from build123d import *

# Parameters (mm, degrees)
F0_W     = 61
F0_H     = 42
F0_W_2   = 28
F0_H_2   = 3.6
F0_R     = 6.5
F0_R_2   = 13.35
F0_R_3   = 11.75
F1_DEPTH = 1.2
F2_DEPTH = 10
F3_DEPTH = 5
F4_W     = 22.4
F4_H     = 2.5
F5_DEPTH = 5


with BuildPart() as f1:
    # F0 (on Top) → F1 (new body)
    with BuildSketch(Plane.XY):
        with Locations((30.5, 21)):
            Rectangle(F0_W, F0_H)
        with Locations((24, 7.8)):
            Rectangle(F0_W_2, F0_H_2, mode=Mode.SUBTRACT)
        with Locations((12.5, 28.3)):
            Circle(F0_R, mode=Mode.SUBTRACT)
        with Locations((44.25, 26.15)):
            Circle(F0_R_2, mode=Mode.SUBTRACT)
        with Locations((44.25, 26.15)):
            Circle(F0_R_2)
        with Locations((44.25, 26.15)):
            Circle(F0_R_3, mode=Mode.SUBTRACT)
    extrude(amount=F1_DEPTH)

    # F0 (on Top) → F2 (join)
    with BuildSketch(Plane.XY):
        with Locations((44.25, 26.15)):
            Circle(F0_R_2)
        with Locations((44.25, 26.15)):
            Circle(F0_R_3, mode=Mode.SUBTRACT)
    extrude(amount=F2_DEPTH)

    # F0 (on Top) → F3 (join)
    with BuildSketch(Plane.XY):
        with Locations((24, 7.8)):
            Rectangle(F0_W_2, F0_H_2)
    extrude(amount=F3_DEPTH)

    # F4 (on face) → F5 (cut)
    with BuildSketch(Plane.XZ.offset(-6)):
        with Locations((24, 2.45)):
            Rectangle(F4_W, F4_H)
    extrude(amount=-F5_DEPTH, mode=Mode.SUBTRACT)


solid = f1.part
Geometry check sheet. Reference: the model listing, model coordinates, mm. A direction names the side the tool comes from. Give positions to 0.01 mm unless a question says otherwise; leave off trailing zeros. Write each loop counter-clockwise with the first axis right and the second up, starting at its lowest first coordinate (ties: lowest second). Pieces come first, ordered by that corner, then holes. Notation, with made-up numbers: M -39.75,39.5 L -24.75,39.5 A10 cw -24.75,44.5 Z; hole C 34.25,-37.75 d7. An arc over 180 degrees is marked long. Answer as CSV lines item,"result". Start each with the question number.
Q1. Section check D-D, the plane x = 14. Record the cut outline in (y, z).
Q2. Tool access check on faces 1 (the face through (56.984, 30.16, 5.538)), 2 (the face through (24, 8, 3.7)), 3 (the face through (12.8, 8, 2)), 4 (the face through (24, 8, 5)). Record the directions out of +Z, -Z, +X, -X, +Y, -Y that give a thin tool (end or side, any length) a straight path to the whole face; none if there is none.
Q3. Section check C-C, the plane z = 8. Record the cut outline in (x, y), then the cut area to 3 significant figures.
Q4. Section check A-A, the plane y = 28.3. Record the cut outline in (x, z).
Q5. Release check for a two-part mould opening along Y. For faces 5 (the face through (32.51, 26.67, 4.93)), 6 (the face through (30, 21, 0)), 7 (the face through (30, 0, 1)) record: pulls with the +Y half, pulls with the -Y half, needs draft (parallel to the pull), parting line crosses it, or undercut.
Q6. Go/stop test with flat-tipped pins: pin 1 (1.5 mm diameter, centred on y = 14, z = 7.5, fed in from -X); pin 2 (15 mm diameter, centred on x = 12.5, y = 28.3, fed in from +Z); pin 3 (14 mm diameter, centred on x = 44.25, y = 26.15, fed in from -Z); pin 4 (3 mm diameter, centred on x = 20, z = 4, fed in from -Y). Record where each tip stops, or that it passes through.
Q7. Section check B-B, the plane x = 44.25. Record the cut outline in (y, z).
Q8. Material ranges on L1, parallel to Y at x = 12.5, z = 0.8; L2, parallel to Z at x = 14.5, y = 7.5; L3, parallel to Y at x = 44, z = 8.25, recorded low to high.
Geometry says:
1,outline,"M 0,0 L 21.98,0 L 21.98,1.2 L 0,1.2 Z; M 6,3.7 L 9.6,3.7 L 9.6,5 L 6,5 Z; M 34.62,0 L 42,0 L 42,1.2 L 34.62,1.2 Z"
2,face 1,"+Z"
2,face 2,"-Y"
2,face 3,"+Y, -Y"
2,face 4,"+Z, +X, -X, -Y"
3,outline,"C 44.25,26.15 d26.7; hole C 44.25,26.15 d23.5"
3,area,"126 mm^2"
4,outline,"M 0,0 L 6,0 L 6,1.2 L 0,1.2 Z; M 19,0 L 32.7,0 L 32.7,10 L 31.07,10 L 31.07,1.2 L 19,1.2 Z; M 55.8,0 L 61,0 L 61,1.2 L 57.43,1.2 L 57.43,10 L 55.8,10 Z"
5,face 5,"undercut"
5,face 6,"needs draft"
5,face 7,"pulls with the -Y half"
6,pin 1,"x = 37.3"
6,pin 2,"z = 1.2"
6,pin 3,"through"
6,pin 4,"y = 6"
7,outline,"M 0,0 L 14.4,0 L 14.4,10 L 12.8,10 L 12.8,1.2 L 0,1.2 Z; M 37.9,0 L 42,0 L 42,1.2 L 39.5,1.2 L 39.5,10 L 37.9,10 Z"
8,L1,"0 to 21.8, 34.8 to 42"
8,L2,"0 to 1.2, 3.7 to 5"
8,L3,"12.8 to 14.4, 37.9 to 39.5"
